```python
from build123d import *

# Parameters (mm, degrees)
F1_DEPTH       = 12.7
F3_R           = 25.4
F3_W           = 12.7
F3_H           = 25.4
F2_R           = 25.4
F2_W           = 12.7
F2_H           = 25.4
F4_DEPTH       = 3.81
F6_D           = 2.7051
F6_DEPTH       = 15.08125
F6_CSINK_D     = 7.7978
F6_CSINK_ANGLE = 82
F6_TIP         = 0.8126940303
F8_D           = 2.7051
F8_DEPTH       = 15.0876
F8_CSINK_D     = 7.7978
F8_CSINK_ANGLE = 82
F8_TIP         = 0.8126940303


with BuildPart() as f1:
    # F0 (on Top) → F1 (new body, symmetric)
    with BuildSketch(Plane.XY):
        Polygon((41.275, 0), (-41.275, 0), (-41.275, 38.1), (-53.975, 38.1), (-53.975, -12.7), (53.975, -12.7), (53.975, 38.1), (41.275, 38.1), align=None)
    extrude(amount=F1_DEPTH, both=True)

    # F3 (on face) + F2 (on face) → F4 (join)
    with BuildSketch(Plane(origin=(0, 38.1, 0), x_dir=(-1, 0, 0), z_dir=(0, 1, 0))):
        with Locations((47.625, 0)):
            Circle(F3_R)
        with Locations((47.625, 0)):
            Rectangle(F3_W, F3_H, mode=Mode.SUBTRACT)
        with Locations((47.625, 0)):
            Rectangle(F3_W, F3_H)
    with BuildSketch(Plane(origin=(0, 38.1, 0), x_dir=(-1, 0, 0), z_dir=(0, 1, 0))):
        with Locations((-47.625, 0)):
            Circle(F2_R)
        with Locations((-47.625, 0)):
            Rectangle(F2_W, F2_H, mode=Mode.SUBTRACT)
        with Locations((-47.625, 0)):
            Rectangle(F2_W, F2_H)
    extrude(amount=F4_DEPTH)

    # F6
    with Locations(Plane(origin=(0, 41.91, 0), x_dir=(-1, 0, 0), z_dir=(0, 1, 0))):
        with Locations((-47.625, 0)):
            CounterSinkHole(F6_D / 2, F6_CSINK_D / 2, depth=F6_DEPTH, counter_sink_angle=F6_CSINK_ANGLE)
            with Locations((0, 0, -(F6_DEPTH + F6_TIP / 2))):  # 118° drill point
                Cone(0, F6_D / 2, F6_TIP, mode=Mode.SUBTRACT)

    # F8
    with Locations(Plane(origin=(0, 41.91, 0), x_dir=(-1, 0, 0), z_dir=(0, 1, 0))):
        with Locations((47.625, 0)):
            CounterSinkHole(F8_D / 2, F8_CSINK_D / 2, depth=F8_DEPTH, counter_sink_angle=F8_CSINK_ANGLE)
            with Locations((0, 0, -(F8_DEPTH + F8_TIP / 2))):  # 118° drill point
                Cone(0, F8_D / 2, F8_TIP, mode=Mode.SUBTRACT)


solid = f1.part
```
The model under review builds one solid part; all positions refer to its coordinate system, in mm. A direction names the side the tool comes from. Round coordinates to 2 decimals unless told otherwise and drop trailing zeros. Loops run counter-clockwise (first coordinate to the right, second up) from the corner with the lowest first, then second, coordinate; pieces in that order, holes last.
1) Consider section C-C on x = 3. State the section outline as (y, z) points, then the cut area to 3 significant figures.
Values follow:
outline: (-12.7, -12.7) - (0, -12.7) - (0, 12.7) - (-12.7, 12.7) - close
area: 323 mm2
2) The part is to be moulded in two halves that separate along X. For faces 5 (the face through (-53.975, 13, 0)), 6 (the face through (53.975, 12, 0)), 7 (the face through (-53, 41.91, 0)), 8 (the face through (-46.335, 32.816, 0.406)), say which applies: pulls with the +X half, pulls with the -X half, needs draft (parallel to the pull), parting line crosses it, or undercut.
Values follow:
face 5: pulls with the -X half
face 6: pulls with the +X half
face 7: needs draft
face 8: undercut
3) Consider section B-B on z = -16. State the section outline as (x, y) points.
Values follow:
outline: (-67.35, 38.1) - (-27.9, 38.1) - (-27.9, 41.91) - (-67.35, 41.91) - close; (27.9, 38.1) - (67.35, 38.1) - (67.35, 41.91) - (27.9, 41.91) - close
4) Clearance check with flat-ended pins moving along their axes: P1, Ø20.5, axis at y = 10.5, z = -6, coming from the -X side (3 decimals); P2, Ø4, axis at x = -16, z = -7.5, coming from the +Y side; P3, Ø12.5, axis at y = 15, z = -4.5, coming from the +X side (3 decimals). State where each tip first meets the part, or that it passes through.
Values follow:
P1: stops at x = -53.975
P2: stops at y = 0
P3: stops at x = 53.975
5) Consider section A-A on y = 36.5. State the section outline as (x, z) points (3 decimals), then the cut area to 3 significant figures.
Values follow:
outline: (-53.975, -12.7) - (-41.275, -12.7) - (-41.275, 12.7) - (-53.975, 12.7) - close; (41.275, -12.7) - (53.975, -12.7) - (53.975, 12.7) - (41.275, 12.7) - close; hole circle Ø2.705 at (-47.625, 0); hole circle Ø2.705 at (47.625, 0)
area: 634 mm2
6) Consider section D-D on z = -6. State the section outline as (x, y) points (3 decimals), then the cut area to 3 significant figures.
Values follow:
outline: (-72.306, 38.1) - (-53.975, 38.1) - (-53.975, -12.7) - (53.975, -12.7) - (53.975, 38.1) - (72.306, 38.1) - (72.306, 41.91) - (22.944, 41.91) - (22.944, 38.1) - (41.275, 38.1) - (41.275, 0) - (-41.275, 0) - (-41.275, 38.1) - (-22.944, 38.1) - (-22.944, 41.91) - (-72.306, 41.91) - close
area: 2,710 mm2
7) Wall thickness on line 1 along X through (y, z) = (36.25, 0) (3 decimals); line 2 along Y through (x, z) = (-23, -1.5); line 3 along Z through (x, y) = (9, -9): over which ranges is each line inside the solid? List them lowest first.
Values follow:
line 1: x = -53.975 to -48.978, -46.272 to -41.275, 41.275 to 46.272, 48.978 to 53.975
line 2: y = -12.7 to 0, 38.1 to 41.91
line 3: z = -12.7 to 12.7
8) Tool access review of faces 1 (the face through (48.915, 32.82, 0.406)), 2 (the face through (-1, -4, -12.7)), 3 (the face through (1, 0, 0)), 4 (the face through (-59, 38.1, 0)): name each direction out of +Z, -Z, +X, -X, +Y, -Y from which nothing blocks a thin tool from reaching the whole face with its end or side.
Values follow:
face 1: +Y
face 2: -Z, +X, -X, -Y
face 3: +Z, -Z
face 4: none
